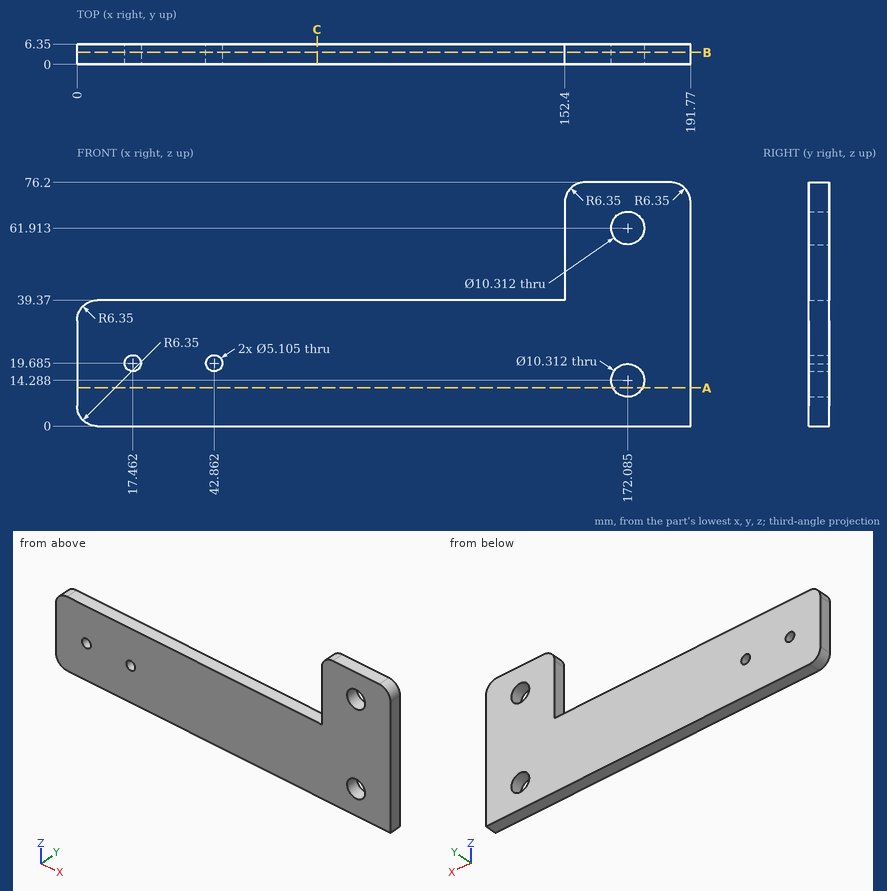
Job drawing, mm, ordinate dimensions from the low corner. One solid piece. Coordinates: 2 decimals unless noted, no trailing zeros. Loops run counter-clockwise (first coordinate to the right, second up) from the corner with the lowest first, then second, coordinate; pieces in that order, holes last. Notation, with made-up numbers: (-33.5, 35.5) -> (9.5, 35.5) arc R14 ccw to (9.5, 50.5) -> close; hole circle Ø9 at (0.5, 79.25). An arc over 180 degrees is marked (long way). One line per item, written item: value.
1. Slice it at C-C on x = 75. Write the cut outline in (y, z).
Answers:
outline: (0, 0) -> (6.35, 0) -> (6.35, 39.37) -> (0, 39.37) -> close
2. Drill centre lines: line 1 (X direction, y = 5, z = 20) (1 decimal); line 2 (X direction, y = 2, z = 19) (1 decimal); line 3 (Z direction, x = 121.5, y = 1). Where is each one in solid material? Low to high. Write a range as [from, to].
Answers:
line 1: x = [0, 14.9], [20, 40.3], [45.4, 191.8]
line 2: x = [0, 15], [19.9, 40.4], [45.3, 170], [174.2, 191.8]
line 3: z = [0, 39.37]
3. Slice it at B-B on y = 3.75. Give the number of separate pieces and of enclosed holes in the cut face, and give its area (3 significant figures).
Answers:
separate pieces: 1
enclosed holes: 4
area: 8,760 mm^2
4. Flat gauge pin, fed straight in: P1, Ø13.5, axis at x = 172.08, z = 61.91, coming from the -Y side. Where does the tip first touch, or does it go through?
Answers:
P1: stops at y = 0
5. Slice it at A-A on z = 12. Write the cut outline in (x, y), and give its area (3 significant figures).
Answers:
outline: (0, 0) -> (167.46, 0) -> (167.46, 6.35) -> (0, 6.35) -> close; (176.71, 0) -> (191.77, 0) -> (191.77, 6.35) -> (176.71, 6.35) -> close
area: 1,160 mm^2
